```python
from build123d import *

# Parameters (mm, degrees)
F0_W     = 101.6
F0_H     = 63.5
F1_DEPTH = 31.75
F2_T     = -4.7625
F4_W     = 53.9496
F4_H     = 22.1996
F6_DEPTH = 1.27
F3_W     = 92.0496
F3_H     = 22.1996
F7_DEPTH = 1.27
F5_W     = 53.9496
F5_H     = 22.1996
F8_DEPTH = 1.27


with BuildPart() as f1:
    # F0 (on Top) → F1 (new body)
    with BuildSketch(Plane.XY):
        Rectangle(F0_W, F0_H)
    extrude(amount=F1_DEPTH)

    # F2
    f2_openings = [f1.faces().sort_by_distance(p)[0] for p in [
        (0, 0, 31.75),
    ]]
    offset(amount=F2_T, openings=f2_openings)

    # F4 (on face) → F6 (cut)
    with BuildSketch(Plane.YZ.offset(50.8)):
        with Locations((0, 15.875)):
            Rectangle(F4_W, F4_H)
    extrude(amount=-F6_DEPTH, mode=Mode.SUBTRACT)

    # F3 (on face) → F7 (cut)
    with BuildSketch(Plane.XZ.offset(31.75)):
        with Locations((0, 15.875)):
            Rectangle(F3_W, F3_H)
    extrude(amount=-F7_DEPTH, mode=Mode.SUBTRACT)

    # F5 (on face) → F8 (cut)
    with BuildSketch(Plane(origin=(-50.8, 0, 0), x_dir=(0, -1, 0), z_dir=(-1, 0, 0))):
        with Locations((0, 15.875)):
            Rectangle(F5_W, F5_H)
    extrude(amount=-F8_DEPTH, mode=Mode.SUBTRACT)


solid = f1.part
```
Build history of the part. All positions in model axes, mm. A direction names the side the tool comes from. Give positions to 0.01 mm unless a question says otherwise; leave off trailing zeros. Loops run counter-clockwise (first coordinate to the right, second up) from the corner with the lowest first, then second, coordinate; pieces in that order, holes last.
Item 1: Which spindle directions (+Z, -Z, +X, -X, +Y, -Y) get a long thin tool onto all of the face, cutting with end or side? Do faces 1 (the face through (-1, 0, 4.762)), 2 (the face through (49.53, 0, 16)), 3 (the face through (-1, -30.48, 16)). Say none if no direction does.
Answers follow:
face 1: +Z
face 2: +X
face 3: -Y
Item 2: Slice it at D-D, the plane z = 19. List the corners of the cut face in (x, y).
Answers follow:
outline: (-50.8, -31.75) - (-46.02, -31.75) - (-46.02, -30.48) - (46.02, -30.48) - (46.02, -31.75) - (50.8, -31.75) - (50.8, -26.97) - (49.53, -26.97) - (49.53, 26.97) - (50.8, 26.97) - (50.8, 31.75) - (-50.8, 31.75) - (-50.8, 26.97) - (-49.53, 26.97) - (-49.53, -26.97) - (-50.8, -26.97) - close; hole (-46.04, -26.99) - (46.04, -26.99) - (46.04, 26.99) - (-46.04, 26.99) - close
Item 3: Drill centre lines: line 1 (X direction, y = -20, z = 21); line 2 (Y direction, x = -12.5, z = 19); line 3 (Y direction, x = 27, z = 27.5). Where is each one in solid material? Low to high.
Answers follow:
line 1: x = -49.53 to -46.04, 46.04 to 49.53
line 2: y = -30.48 to -26.99, 26.99 to 31.75
line 3: y = -31.75 to -26.99, 26.99 to 31.75
Item 4: Flat gauge pins, fed straight in: pin 1 (1 mm diameter, centred on y = -24.5, z = 14.5, fed in from -X); pin 2 (4 mm diameter, centred on x = -15, z = 9, fed in from -Y). Where does each tip first touch, or does it go through?
Answers follow:
pin 1: stops at x = -49.53
pin 2: stops at y = -30.48
Item 5: Slice it at C-C, the plane y = -11. List the corners of the cut face in (x, z), and give its area (3 significant figures).
Answers follow:
outline: (-50.8, 0) - (50.8, 0) - (50.8, 4.78) - (49.53, 4.78) - (49.53, 26.97) - (50.8, 26.97) - (50.8, 31.75) - (46.04, 31.75) - (46.04, 4.76) - (-46.04, 4.76) - (-46.04, 31.75) - (-50.8, 31.75) - (-50.8, 26.97) - (-49.53, 26.97) - (-49.53, 4.78) - (-50.8, 4.78) - close
area: 685 mm2
Item 6: Slice it at B-B, the plane x = 9.5. List the corners of the cut face in (y, z), and give its area (3 significant figures).
Answers follow:
outline: (-31.75, 0) - (31.75, 0) - (31.75, 31.75) - (26.99, 31.75) - (26.99, 4.76) - (-26.99, 4.76) - (-26.99, 31.75) - (-31.75, 31.75) - (-31.75, 26.97) - (-30.48, 26.97) - (-30.48, 4.78) - (-31.75, 4.78) - close
area: 531 mm2
Item 7: Slice it at A-A, the plane z = 28.5. List the corners of the cut face in (x, y).
Answers follow:
outline: (-50.8, -31.75) - (50.8, -31.75) - (50.8, 31.75) - (-50.8, 31.75) - close; hole (-46.04, -26.99) - (46.04, -26.99) - (46.04, 26.99) - (-46.04, 26.99) - close
Item 8: Pull direction X, two halves, no side cores. Call faces 4 (the face through (46.037, 0, 18)), 5 (the face through (-1, 0, 0)), 6 (the face through (-50.8, 0, 30)): released by +X, released by -X, zero draft, split by the parting line, or undercut.
Answers follow:
face 4: undercut
face 5: zero draft
face 6: released by -X
